CAD build for the part. Positions are in the model's coordinates, mm. Round coordinates to 2 decimals unless told otherwise and drop trailing zeros. Loops run counter-clockwise (first coordinate to the right, second up) from the corner with the lowest first, then second, coordinate; pieces in that order, holes last. Notation, with made-up numbers: M 29.25,51 L 42.25,51 A19 ccw 42.25,58 Z; hole C 10,47.5 d2. An arc over 180 degrees is marked long. Use one line per item in the form item = value.
from build123d import *

# Parameters (mm, degrees)
SKETCH1_W           = 50.8
SKETCH1_H           = 50.8
BOSS_EXTRUDE1_DEPTH = 50.8
FILLET1_R           = 3.175
SKETCH2_R           = 2.4892
CUT_EXTRUDE1_DEPTH  = 88.988181024


with BuildPart() as part:
    # Sketch1 → Boss-Extrude1 (new body)
    with BuildSketch(Plane.XY):
        with Locations((25.4, 25.4)):
            Rectangle(SKETCH1_W, SKETCH1_H)
    extrude(amount=-BOSS_EXTRUDE1_DEPTH)

    # Fillet1
    fillet1_edges = [part.edges().sort_by_distance(p)[0] for p in [
        (50.8, 25.4, -50.8),
        (25.4, 50.8, -50.8),
        (0, 25.4, -50.8),
        (25.4, 50.8, 0),
        (50.8, 25.4, 0),
        (25.4, 0, 0),
        (0, 25.4, 0),
        (0, 50.8, -25.4),
        (50.8, 50.8, -25.4),
        (50.8, 0, -25.4),
        (0, 0, -25.4),
        (25.4, 0, -50.8),
    ]]
    fillet(fillet1_edges, radius=FILLET1_R)

    # Sketch2 → Cut-Extrude1 (cut, through all)
    with BuildSketch(Plane.ZY):
        with Locations((-38.1, 12.7)):
            Circle(SKETCH2_R)
        with Locations((-12.7, 12.7)):
            Circle(SKETCH2_R)
        with Locations((-12.7, 38.1)):
            Circle(SKETCH2_R)
        with Locations((-38.1, 38.1)):
            Circle(SKETCH2_R)
    extrude(amount=-CUT_EXTRUDE1_DEPTH, mode=Mode.SUBTRACT)


solid = part.part
1. Cut at C-C on x = 24. Write the cut outline in (y, z) (3 decimals), and give its area (3 significant figures).
Completed:
outline = M 0,-47.625 A3.175 ccw 3.175,-50.8 L 47.625,-50.8 A3.175 ccw 50.8,-47.625 L 50.8,-3.175 A3.175 ccw 47.625,0 L 3.175,0 A3.175 ccw 0,-3.175 Z; hole C 12.7,-38.1 d4.978; hole C 12.7,-12.7 d4.978; hole C 38.1,-38.1 d4.978; hole C 38.1,-12.7 d4.978
area = 2,490 mm2
2. Cut at A-A on z = -12.7. Write the cut outline in (x, y) (3 decimals), and give its area (3 significant figures).
Completed:
outline = M 0,3.175 A3.175 ccw 3.175,0 L 47.625,0 A3.175 ccw 50.8,3.175 L 50.8,10.211 L 0,10.211 Z; M 0,15.189 L 50.8,15.189 L 50.8,35.611 L 0,35.611 Z; M 0,40.589 L 50.8,40.589 L 50.8,47.625 A3.175 ccw 47.625,50.8 L 3.175,50.8 A3.175 ccw 0,47.625 Z
area = 2,070 mm2
3. Cut at B-B on y = 38.1. Write the cut outline in (x, z) (3 decimals), and give its area (3 significant figures).
Completed:
outline = M 0,-47.625 A3.175 ccw 3.175,-50.8 L 47.625,-50.8 A3.175 ccw 50.8,-47.625 L 50.8,-40.589 L 0,-40.589 Z; M 0,-35.611 L 50.8,-35.611 L 50.8,-15.189 L 0,-15.189 Z; M 0,-10.211 L 50.8,-10.211 L 50.8,-3.175 A3.175 ccw 47.625,0 L 3.175,0 A3.175 ccw 0,-3.175 Z
area = 2,070 mm2
4. Pull direction Y, two halves, no side cores. Call faces 1 (the face through (25, 0, -25)), 2 (the face through (25.044, 35.892, -11.551)), 3 (the face through (0.91, 25.71, -0.95)), 4 (the face through (25.04, 14.8, -11.36)): +Y half, -Y half, draft (parallel to the pull), parting line (faces both ways), or undercut.
Completed:
face_1 = -Y half
face_2 = undercut
face_3 = draft
face_4 = undercut
5. Drop a flat-ended pin along its axis: P1, Ø5, axis at y = 10.5, z = -14.5, coming from the -X side. Give the stop position or say it passes through.
Completed:
P1 = 0
6. Probe line 1 along Y through (x, z) = (17, -12.7); line 2 along Y through (x, z) = (13.5, -39.5); line 3 along Z through (x, y) = (22, 14). List the from-to ranges inside material, lowest first. Write a range as from..to.
Completed:
line_1 = 0..10.21, 15.19..35.61, 40.59..50.8
line_2 = 0..10.64, 14.76..36.04, 40.16..50.8
line_3 = -50.8..-40.22, -35.98..-14.82, -10.58..0
